Verification items for the finished model (mm, model axes). Coordinates: 2 decimals unless noted, no trailing zeros. Loops run counter-clockwise (first coordinate to the right, second up) from the corner with the lowest first, then second, coordinate; pieces in that order, holes last.
Q1. Material ranges on probe 1 along Y at (x, z) = (21, -7); probe 2 along X at (y, z) = (9.25, -3.5); probe 3 along Z at (x, y) = (17.5, 3.75), recorded low to high.
Q2. Sectioned sample at B-B (y = 2.5). Enter the section's corners in (x, z).
Q3. Sectioned sample at D-D (y = 12.5). Enter the section's corners in (x, z), then the cut area to 3 significant figures.
Q4. Go/stop test with flat-tipped pins: P1, Ø0.8, axis at y = 2.5, z = -7, coming from the +X side; P2, Ø0.9, axis at y = 4.5, z = -7, coming from the -X side. Record where each tip stops, or that it passes through.
Q5. Sectioned sample at C-C (z = -7). Enter the section's corners in (x, y), then the cut area to 3 significant figures.
Q6. Sectioned sample at A-A (x = 3.25). Enter the section's corners in (y, z), then the cut area to 3 significant figures.
```python
from build123d import *

# Parameters (mm, degrees)
SKETCH1_W           = 25
SKETCH1_H           = 10
BOSS_EXTRUDE1_DEPTH = 15
SKETCH2_R           = 0.75
CUT_EXTRUDE1_DEPTH  = 10
SKETCH3_R           = 0.75
CUT_EXTRUDE2_DEPTH  = 10
SKETCH4_R           = 0.75
CUT_EXTRUDE3_DEPTH  = 10


with BuildPart() as part:
    # Sketch1 → Boss-Extrude1 (new body)
    with BuildSketch(Plane(origin=(0, 0, 0), x_dir=(1, 0, 0), z_dir=(0, 1, 0))):
        with Locations((12.5, 5)):
            Rectangle(SKETCH1_W, SKETCH1_H)
    extrude(amount=BOSS_EXTRUDE1_DEPTH)

    # Sketch2 → Cut-Extrude1 (cut)
    with BuildSketch(Plane.XZ):
        with Locations((7.5, -4)):
            Circle(SKETCH2_R)
        with Locations((17.5, -4)):
            Circle(SKETCH2_R)
    extrude(amount=-CUT_EXTRUDE1_DEPTH, mode=Mode.SUBTRACT)

    # Sketch3 → Cut-Extrude2 (cut)
    with BuildSketch(Plane.ZY):
        with Locations((-7, 10.5)):
            Circle(SKETCH3_R)
        with Locations((-7, 4.5)):
            Circle(SKETCH3_R)
    extrude(amount=-CUT_EXTRUDE2_DEPTH, mode=Mode.SUBTRACT)

    # Sketch4 → Cut-Extrude3 (cut)
    with BuildSketch(Plane(origin=(25, 0, 0), x_dir=(0, 0, -1), z_dir=(1, 0, 0))):
        with Locations((7, 12.5)):
            Circle(SKETCH4_R)
        with Locations((7, 2.5)):
            Circle(SKETCH4_R)
    extrude(amount=-CUT_EXTRUDE3_DEPTH, mode=Mode.SUBTRACT)


solid = part.part
```
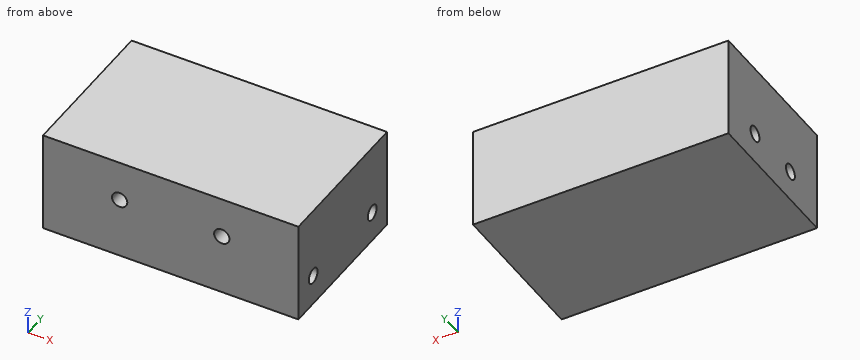
Geometry check:
1. probe 1: y = 0 to 1.75, 3.25 to 11.75, 13.25 to 15
1. probe 2: x = 0 to 6.94, 8.06 to 16.94, 18.06 to 25
1. probe 3: z = -10 to -4.75, -3.25 to 0
2. outline: (0, -10) - (25, -10) - (25, -7.75) - (15, -7.75) - (15, -6.25) - (25, -6.25) - (25, 0) - (0, 0) - close; hole circle Ø1.5 at (7.5, -4); hole circle Ø1.5 at (17.5, -4)
3. outline: (0, -10) - (25, -10) - (25, -7.75) - (15, -7.75) - (15, -6.25) - (25, -6.25) - (25, 0) - (0, 0) - close
3. area: 235 mm2
4. P1: stops at x = 15
4. P2: stops at x = 10
5. outline: (0, 0) - (25, 0) - (25, 1.75) - (15, 1.75) - (15, 3.25) - (25, 3.25) - (25, 11.75) - (15, 11.75) - (15, 13.25) - (25, 13.25) - (25, 15) - (0, 15) - (0, 11.25) - (10, 11.25) - (10, 9.75) - (0, 9.75) - (0, 5.25) - (10, 5.25) - (10, 3.75) - (0, 3.75) - close
5. area: 315 mm2
6. outline: (0, -10) - (15, -10) - (15, 0) - (0, 0) - close; hole circle Ø1.5 at (4.5, -7); hole circle Ø1.5 at (10.5, -7)
6. area: 146 mm2
